Geometry check sheet. Reference: the model listing, model coordinates, mm. A direction names the side the tool comes from. Coordinates: 2 decimals unless noted, no trailing zeros. Loops run counter-clockwise (first coordinate to the right, second up) from the corner with the lowest first, then second, coordinate; pieces in that order, holes last. Notation, with made-up numbers: M 56,-10 L 111,-10 A21 ccw 111,-5 Z; hole C 54,85 d7. An arc over 180 degrees is marked long. One line per question, with ' | ' between items. Start each with the question number.
from build123d import *

# Parameters (mm, degrees)
F1_DEPTH = 25.4
F2_W     = 41.815902
F2_H     = 7.212999
F3_DEPTH = 25.4
F5_DEPTH = 7.62
F6_R     = 2.506654
F7_DEPTH = 45.974


with BuildPart() as f1:
    # F0 (on Front) → F1 (new body)
    with BuildSketch(Plane.XZ):
        with BuildLine():
            Line((75.069629, 11.929201), (-75.792603, 11.929201))
            Line((-75.792603, 11.929201), (-75.792603, 9.196899))
            ThreePointArc((-75.792603, 9.196899), (-73.507023, 8.250181), (-72.560304, 5.9646))
            ThreePointArc((-72.560304, 5.9646), (-73.507023, 3.67902), (-75.792603, 2.732302))
            Line((-75.792603, 2.732302), (-75.792603, 0))
            Line((-75.792603, 0), (75.069629, 0))
            Line((75.069629, 0), (75.069629, 2.7388))
            ThreePointArc((75.069629, 2.7388), (71.843829, 5.9646), (75.069629, 9.1904))
            Line((75.069629, 9.1904), (75.069629, 11.929201))
        make_face()
        with BuildLine():
            Line((-75.792603, 9.196899), (-75.792603, 11.929201))
            ThreePointArc((-75.792603, 11.929201), (-81.757204, 5.9646), (-75.792603, 0))
            Line((-75.792603, 0), (-75.792603, 2.732302))
            ThreePointArc((-75.792603, 2.732302), (-79.024902, 5.9646), (-75.792603, 9.196899))
        make_face()
        with BuildLine():
            ThreePointArc((75.069629, 0), (81.034229, 5.9646), (75.069629, 11.929201))
            Line((75.069629, 11.929201), (75.069629, 9.1904))
            ThreePointArc((75.069629, 9.1904), (77.350614, 8.245586), (78.295429, 5.9646))
            ThreePointArc((78.295429, 5.9646), (77.350614, 3.683615), (75.069629, 2.7388))
            Line((75.069629, 2.7388), (75.069629, 0))
        make_face()
    extrude(amount=F1_DEPTH)

    # F2 (on Front) → F3 (join)
    with BuildSketch(Plane.XZ):
        with Locations((4.981325, 6.141954)):
            Rectangle(F2_W, F2_H)
    extrude(amount=-F3_DEPTH)

    # F4 (on face) → F5 (cut)
    with BuildSketch(Plane.XY.offset(9.748454)):
        with BuildLine():
            Line((18.730404, 25.4), (-8.149876, 25.4))
            ThreePointArc((-8.149876, 25.4), (5.290264, 12.121353), (18.730404, 25.4))
        make_face()
    extrude(amount=-F5_DEPTH, mode=Mode.SUBTRACT)

    # F6 (on face) → F7 (cut)
    with BuildSketch(Plane(origin=(-15.926626, 0, 0), x_dir=(0, -1, 0), z_dir=(-1, 0, 0))):
        with Locations((-19.283704, 6.176639)):
            Circle(F6_R)
    extrude(amount=-F7_DEPTH, mode=Mode.SUBTRACT)


solid = f1.part
1. Draft check along Y on faces 1 (the cylindrical face through (-11.709, 16.893, 6.93)), 2 (the cylindrical face through (81.033, -12.522, 5.833)), 3 (the flat face through (-2, -25.4, 6)), 4 (the cylindrical face through (21.762, 16.893, 6.93)). Enter one of: +Y half, -Y half, draft (parallel to the pull), parting line (faces both ways), or undercut.
2. Tool access check on faces 5 (the flat face through (5, 10, 2.535)), 6 (the flat face through (5, 10, 9.748)), 7 (the flat face through (-15.927, 13, 6)). Record the directions out of +Z, -Z, +X, -X, +Y, -Y that give a thin tool (end or side, any length) a straight path to the whole face; none if there is none.
3. Sectioned sample at B-B (y = 14). Record the cut outline in (x, z).
4. Sectioned sample at A-A (y = -16). Record the cut outline in (x, z), and give its area (3 significant figures).
5. Depth check by flat-ended pin: pin 1 Ø3 at (y, z) = (19.28, 6.18) entering from +X; pin 2 Ø2 at (y, z) = (10.5, 7) entering from +X; pin 3 Ø6 at (y, z) = (13.5, 6.5) entering from -X; pin 4 Ø1.5 at (x, z) = (1, 8.5) entering from +Y. Enter the tip coordinate at first touch or a pass-through.
6. Sectioned sample at C-C (x = -59). Record the cut outline in (y, z), and give its area (3 significant figures).
7. Thickness scan on line 1 (X direction, y = -4, z = 6.25); line 2 (X direction, y = -21, z = 6.5); line 3 (Y direction, x = 50.5, z = 1.25). Record the ranges inside material, lowest first.
Result:
1) face 1: undercut | face 2: draft | face 3: -Y half | face 4: undercut
2) face 5: -Z, +X, -X, +Y | face 6: +Z, +X, -X, +Y | face 7: +Z, -Z, -X, +Y
3) outline: M -15.93,2.54 L -1.56,2.54 L -1.56,9.75 L -15.93,9.75 Z; M 12.14,2.54 L 25.89,2.54 L 25.89,9.75 L 12.14,9.75 Z
4) outline: M -75.79,0 L 75.07,0 A5.96 ccw 75.07,11.93 L -75.79,11.93 A5.96 ccw Z; hole M -75.79,2.73 A3.23 ccw -72.56,5.96 A3.23 ccw long Z; hole M 75.07,9.19 A3.23 ccw long 78.3,5.96 A3.23 ccw Z | area: 1,850 mm2
5) pin 1: passes through | pin 2: stops at x = 25.89 | pin 3: stops at x = -15.93 | pin 4: stops at y = 13.1
6) outline: M -25.4,0 L 0,0 L 0,11.93 L -25.4,11.93 Z | area: 303 mm2
7) line 1: x = -81.75 to -79.01, -72.57 to 71.86, 78.28 to 81.03 | line 2: x = -81.73 to -78.98, -72.6 to 71.89, 78.25 to 81.01 | line 3: y = -25.4 to 0
